For this review, take the finished solid that the model builds, in its own axes (mm). A direction names the side the tool comes from. Give positions to 0.01 mm unless a question says otherwise; leave off trailing zeros. Order: outer loops, then holes, each group sorted by start corner. A loop starts at its lowest first (then second) coordinate and runs counter-clockwise, first axis right, second up.
Item 1: Consider section A-A (y = 1.27). Give the boundary of the cut face in (x, z) (3 decimals).
Item 2: Consider section D-D (z = -4). Give the boundary of the cut face in (x, y).
Item 3: For probe 1 along Z at (x, y) = (8.25, 1.27) (3 decimals); probe 2 along Y at (x, z) = (-9, 21.5); probe 3 along Z at (x, y) = (19.5, 2.5), list the stretches that pass through material, from the lowest coordinate up.
Item 4: Machinability: for faces 4 (the flat face through (0, 2.54, 2)), 5 (the flat face through (0, 0, 2)), 6 (the flat face through (-19, 1, -17.706)), 7 (the flat face through (-5.08, -1, -22)), 8 (the flat face through (19, 1, -17.706)), which of the approach directions +Z, -Z, +X, -X, +Y, -Y give a long, thin tool a straight path to every point of the face, cutting with its end or side? Answer none if there is none.
Item 5: Consider section C-C (x = -8). Give the boundary of the cut face in (y, z), plus the area to 3 significant figures.
Item 6: For P1, Ø2.5, axis at y = 2.5, z = -24, coming from the -X side; P2, Ø12, axis at x = 13.5, z = -22.5, coming from the -Y side; P3, Ø1.3, axis at x = 1.5, y = 1.5, coming from the -Z side; P4, Ø4.5, axis at y = 2, z = -22, coming from the +X side, all flat-tipped, find the tip position at first contact; note any pin that passes through.
Item 7: Consider section B-B (y = 4.75). Give the boundary of the cut face in (x, z).
Item 8: The part is to be moulded in two halves that separate along X. For faces 1 (the flat face through (-23.876, 1, 4)), 2 (the flat face through (0, 1, -17.706)), 3 (the cylindrical face through (9.587, 0.923, -21.994)), say which applies: released by +X, released by -X, zero draft, split by the parting line, or undercut.
```python
from build123d import *

# Parameters (mm, degrees)
SKETCH1_W               = 47.752
SKETCH1_H               = 40.64
BOSS_EXTRUDE1_DEPTH     = 2.54
SKETCH3_R               = 4.572
BOSS_EXTRUDE3_DEPTH     = 23.876
SKETCH7_W               = 10.16
SKETCH7_H               = 13.274102891
SKETCH7_W_2             = 10.953832873
SKETCH7_H_2             = 12.896384516
SKETCH7_W_3             = 11.331551248
CUT_EXTRUDE4_DEPTH      = 47.752
CUT_EXTRUDE4_DEPTH_BACK = 2.54
SKETCH8_W               = 47.752
SKETCH8_H               = 2.54
BOSS_EXTRUDE4_DEPTH     = 5.08
SKETCH9_R               = 2.667
CUT_EXTRUDE5_DEPTH      = 33.782


with BuildPart() as part:
    # Sketch1 → Boss-Extrude1 (new body)
    with BuildSketch(Plane(origin=(0, 0, 0), x_dir=(1, 0, 0), z_dir=(0, 1, 0))):
        Rectangle(SKETCH1_W, SKETCH1_H)
    extrude(amount=BOSS_EXTRUDE1_DEPTH)

    # Sketch3 → Boss-Extrude3 (add, symmetric)
    with BuildSketch(Plane(origin=(0, 0, 0), x_dir=(0, 0, -1), z_dir=(1, 0, 0))):
        with Locations((24.638, 1.27)):
            Circle(SKETCH3_R)
    extrude(amount=BOSS_EXTRUDE3_DEPTH, both=True)

    # Sketch7 → Cut-Extrude4 (cut, two sides)
    with BuildSketch(Plane(origin=(0, 0, -20.245929418), x_dir=(-1, 0, 0), z_dir=(0, 0, -1))) as cut_extrude4_sk:
        with Locations((0, 0.687607575)):
            Rectangle(SKETCH7_W, SKETCH7_H)
        with Locations((19.446916437, 0.498748388)):
            Rectangle(SKETCH7_W_2, SKETCH7_H_2)
        with Locations((-19.635775624, 0.687607575)):
            Rectangle(SKETCH7_W_3, SKETCH7_H)
    extrude(amount=CUT_EXTRUDE4_DEPTH, mode=Mode.SUBTRACT)
    extrude(cut_extrude4_sk.sketch, amount=-CUT_EXTRUDE4_DEPTH_BACK, mode=Mode.SUBTRACT)

    # Sketch8 → Boss-Extrude4 (add)
    with BuildSketch(Plane.XY.offset(20.32)):
        with Locations((0, 1.27)):
            Rectangle(SKETCH8_W, SKETCH8_H)
    extrude(amount=BOSS_EXTRUDE4_DEPTH)

    # Sketch9 → Cut-Extrude5 (cut)
    with BuildSketch(Plane(origin=(13.97, 0, 0), x_dir=(0, 0, -1), z_dir=(1, 0, 0))):
        with Locations(Location((24.638, 1.27, 0), (0, 0, 90))):  # turned: the seam where the file's is
            Circle(SKETCH9_R)
    extrude(amount=-CUT_EXTRUDE5_DEPTH, mode=Mode.SUBTRACT)


solid = part.part
```
Resolved:
1. outline: (-23.876, -17.706) - (-13.97, -17.706) - (-13.97, -21.971) - (-5.08, -21.971) - (-5.08, -17.706) - (5.08, -17.706) - (5.08, -21.971) - (13.97, -21.971) - (13.97, -17.706) - (23.876, -17.706) - (23.876, 25.4) - (-23.876, 25.4) - close; (-13.97, -29.21) - (-5.08, -29.21) - (-5.08, -27.305) - (-13.97, -27.305) - close; (5.08, -29.21) - (13.97, -29.21) - (13.97, -27.305) - (5.08, -27.305) - close
2. outline: (-23.88, 0) - (23.88, 0) - (23.88, 2.54) - (-23.88, 2.54) - close
3. probe 1: z = -29.21 to -27.305, -21.971 to 25.4
3. probe 2: y = 0 to 2.54
3. probe 3: z = -17.71 to 25.4
4. face 4: +Z, +X, -X, +Y
4. face 5: +Z, +X, -X, -Y
4. face 6: -Z, -X, +Y, -Y
4. face 7: -Z, +Y, -Y
4. face 8: -Z, +X, +Y, -Y
5. outline: (0, -20.25) arc R4.57 ccw (long way) to (2.54, -20.25) - (2.54, 25.4) - (0, 25.4) - close; hole circle Ø5.33 at (1.27, -24.64)
5. area: 159 mm2
6. P1: passes through
6. P2: stops at y = -3.3
6. P3: stops at z = -17.71
6. P4: stops at x = 13.97
7. outline: (-13.97, -27.6) - (-5.08, -27.6) - (-5.08, -21.67) - (-13.97, -21.67) - close; (5.08, -27.6) - (13.97, -27.6) - (13.97, -21.67) - (5.08, -21.67) - close
8. face 1: released by -X
8. face 2: undercut
8. face 3: zero draft
